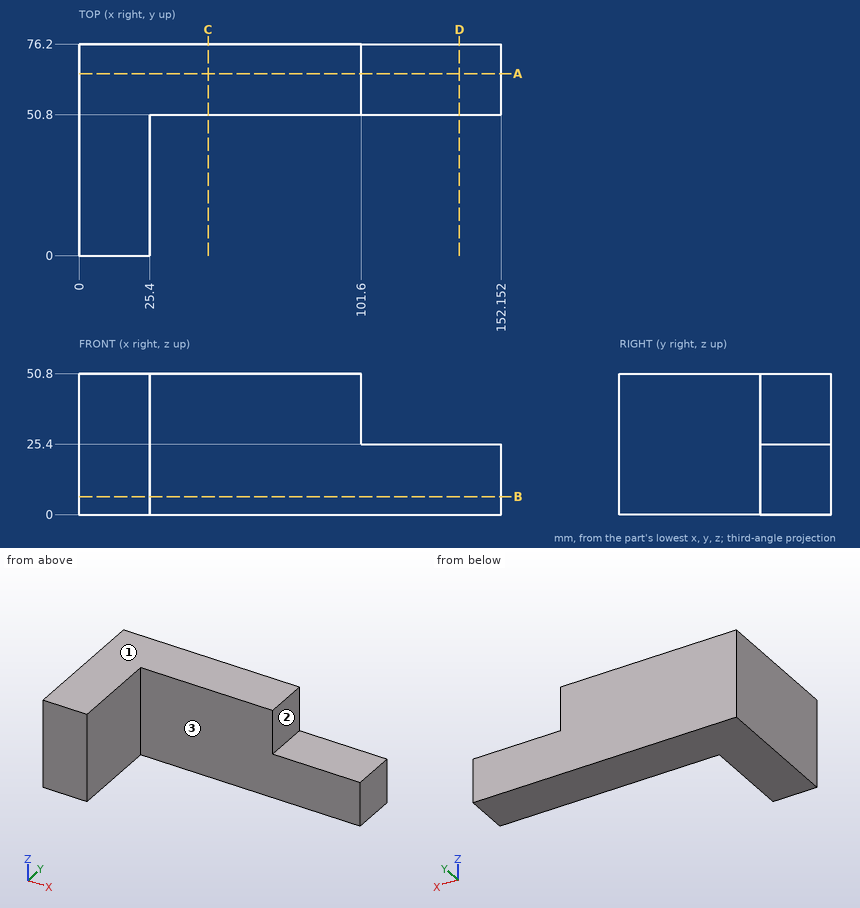
Could you check a few things on this drawing? It's one solid part, dimensions in mm from its lowest x, y, z. A direction names the side the tool comes from. Coordinates: 2 decimals unless noted, no trailing zeros. Order: outer loops, then holes, each group sorted by start corner. A loop starts at its lowest first (then second) coordinate and runs counter-clockwise, first axis right, second up. Notation, with made-up numbers: M 10.25,37 L 52.25,37 A15 cw 52.25,45 Z; hole C 15,3 d4. An arc over 180 degrees is marked long. Use one line per item in the form item = value. Start each with the question number.
1. Suppose I cut it at D-D on x = 137. Write out the boundary of the cut face in (y, z).
2. Please list where these lines run through material, in increasing order: line 1 (X direction, y = 13.5, z = 44); line 2 (Y direction, x = 120, z = 21).
3. Suppose I cut it at C-C on x = 46.5. Write out the boundary of the cut face in (y, z).
4. For pin 1 (1 mm diameter, centred on y = 65, z = 41.5, fed in from +X); pin 2 (20.5 mm diameter, centred on x = 133.5, y = 64.5, fed in from +Z); pin 3 (2 mm diameter, centred on x = 33.5, z = 19, fed in from -Y), each with a flat end and sliding along its axis, tell me the tip position at first contact or that it passes through.
5. Suppose I cut it at A-A on y = 65.5. Write out the boundary of the cut face in (x, z), then the cut area to 3 significant figures.
6. On a 3-axis mill with a long thin cutter (end or side, diameter ignored), from which of +Z, -Z, +X, -X, +Y, -Y can I reach the whole of each face in a straight line? I mean the marked faces 1, 2 and 3. Say none if no direction works.
7. Suppose I cut it at B-B on z = 6.5. Write out the boundary of the cut face in (x, y).
Geometry says:
q1.outline = M 50.8,0 L 76.2,0 L 76.2,25.4 L 50.8,25.4 Z
q2.line_1 = 0 to 25.4
q2.line_2 = 50.8 to 76.2
q3.outline = M 50.8,0 L 76.2,0 L 76.2,50.8 L 50.8,50.8 Z
q4.pin_1 = 101.6
q4.pin_2 = 25.4
q4.pin_3 = 50.8
q5.outline = M 0,0 L 152.15,0 L 152.15,25.4 L 101.6,25.4 L 101.6,50.8 L 0,50.8 Z
q5.area = 6,450 mm^2
q6.face_1 = +Z, +X, -X, +Y, -Y
q6.face_2 = +Z, +X, +Y, -Y
q6.face_3 = +Z, -Z, +X, -Y
q7.outline = M 0,0 L 25.4,0 L 25.4,50.8 L 152.15,50.8 L 152.15,76.2 L 0,76.2 Z
